The model under review builds one solid part; all positions refer to its coordinate system, in mm. Face numbers are marked on the shaded views. Coordinates: 2 decimals unless noted, no trailing zeros. Write each loop counter-clockwise with the first axis right and the second up, starting at its lowest first coordinate (ties: lowest second). Pieces come first, ordered by that corner, then holes. Notation, with made-up numbers: M 10.5,-24.5 L 23.5,-24.5 A28 ccw 23.5,6.5 Z; hole C 17,-18 d1. An arc over 180 degrees is marked long. Answer as a JSON object with one key per item and string values.
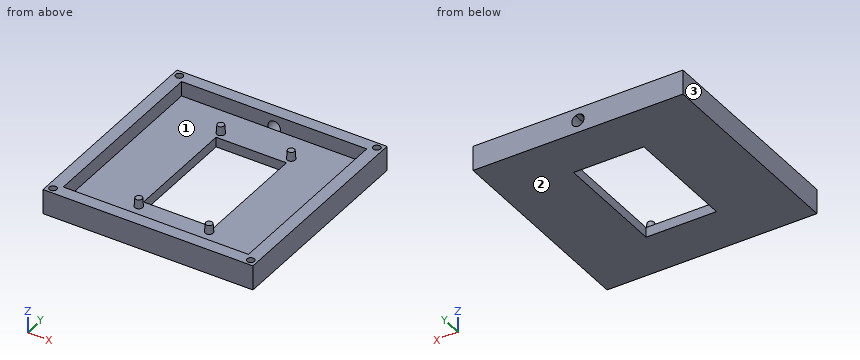
Autodesk Fusion 360 part; units mm, degrees
sketch "Sketch1" plane through (0, 0, 0) normal (0, 0, 1) x (1, 0, 0)
  line L0 (0, 0) -> (0, 75)
  line L1 (0, 75) -> (75, 75)
  line L2 (0, 0) -> (75, 0)
  line L3 (75, 0) -> (75, 75)
  line L4 (75, 75) -> (0, 75)
  line L5 (0, 75) -> (0, 0)
  line L6 (-5, -5) -> (80, -5)
  line L7 (80, -5) -> (80, 80)
  line L8 (80, 80) -> (-5, 80)
  line L9 (-5, 80) -> (-5, -5)
  line L10 (-5, -5) -> (80, -5)
  line L11 (80, -5) -> (80, 80)
  dimension "d1" = 75
  dimension "d2" = 75
  dimension "d3" = 85
extrude "Extrude1" add sketch "Sketch1" along normal blind 10
sketch "Sketch2" plane through (0, 0, 0) normal (0, 0, 1) x (1, 0, 0)
  line L0 (0, 0) -> (75, 0)
  line L1 (75, 0) -> (75, 75)
  line L2 (75, 75) -> (0, 75)
  line L3 (0, 75) -> (0, 0)
extrude "Extrude2" add sketch "Sketch2" along normal blind 4
sketch "Sketch3" plane through (0, 0, 4) normal (0, 0, 1) x (-1, 0, 0)
  line L0 (0, -75) -> (0, 0)
  line L1 (0, 0) -> (-75, 0)
  line L2 (-75, 0) -> (-75, -75)
  line L3 (-75, -75) -> (0, -75)
  line L4 (0, -75) -> (-75, 0)
  line L5 (0, 0) -> (-75, -75)
  line L6 (-37.5, -37.5) -> (-20.25, -37.5)
  line L7 (-37.5, -37.5) -> (-54.75, -37.5)
  line L8 (-20.25, -37.5) -> (-20.25, -66.5)
  line L9 (-54.75, -37.5) -> (-54.75, -8.5)
  line L10 (-20.25, -66.5) -> (-54.75, -66.5)
  line L11 (-54.75, -66.5) -> (-54.75, -8.5)
  line L12 (-54.75, -8.5) -> (-20.25, -8.5)
  line L13 (-20.25, -8.5) -> (-20.25, -66.5)
  line L14 (-37.5, -37.5) -> (-37.5, -60.5)
  line L15 (-37.5, -37.5) -> (-37.5, -14.5)
  line L16 (-37.5, -14.5) -> (-51.75, -14.5)
  line L17 (-37.5, -60.5) -> (-23.25, -60.5)
  line L18 (-23.25, -60.5) -> (-51.75, -60.5)
  line L19 (-51.75, -60.5) -> (-51.75, -14.5)
  line L20 (-51.75, -14.5) -> (-23.25, -14.5)
  line L21 (-23.25, -14.5) -> (-23.25, -60.5)
  dimension "d8" = 17.25
  dimension "d9" = 17.25
  dimension "d10" = 29
  dimension "d11" = 29
  dimension "d12" = 23
  dimension "d13" = 23
  dimension "d14" = 14.25
  dimension "d15" = 14.25
extrude "Extrude3" cut sketch "Sketch3" against normal blind 5 contours L4 L14 L17 L18 L21 | L4 L6 L21 | L5 L6 L21 | L5 L15 L20 L21 | L5 L7 L19 | L5 L14 L18 L19 | L4 L7 L19 | L4 L15 L16 L19 L20
sketch "Sketch4" plane through (0, 0, 4) normal (0, 0, 1) x (-1, 0, 0)
  line L0 (-51.75, -60.5) -> (-51.75, -14.5)
  line L1 (-51.75, -14.5) -> (-23.25, -14.5)
  line L2 (-23.25, -14.5) -> (-23.25, -60.5)
  line L3 (-23.25, -60.5) -> (-51.75, -60.5)
  line L4 (0, -75) -> (0, 0)
  line L5 (0, 0) -> (-75, 0)
  line L6 (-75, 0) -> (-75, -75)
  line L7 (-75, -75) -> (0, -75)
  line L8 (-75, 0) -> (0, -75)
  line L9 (-75, -75) -> (0, 0)
  line L10 (-37.5, -37.5) -> (-54.75, -37.5)
  line L11 (-54.75, -37.5) -> (-54.75, -8.5)
  line L12 (-54.75, -8.5) -> (-20.25, -8.5)
  line L13 (-20.25, -8.5) -> (-20.25, -66.5)
  line L14 (-20.25, -66.5) -> (-54.75, -66.5)
  line L15 (-54.75, -66.5) -> (-54.75, -8.5)
  line L16 (-54.75, -8.5) -> (-20.25, -8.5)
  line L17 (-20.25, -8.5) -> (-20.25, -66.5)
  line L18 (-20.25, -66.5) -> (-20.25, -63.5)
  line L19 (-20.25, -63.5) -> (-23.25, -63.5)
  circle A0 centre (-23.25, -63.5) radius 1.6
  line L20 (-54.75, -66.5) -> (-51.75, -66.5)
  line L21 (-51.75, -66.5) -> (-51.75, -63.5)
  circle A1 centre (-51.75, -63.5) radius 1.6
  line L22 (-20.25, -8.5) -> (-23.25, -8.5)
  line L23 (-23.25, -8.5) -> (-23.25, -11.5)
  circle A2 centre (-23.25, -11.5) radius 1.6
  line L24 (-54.75, -8.5) -> (-54.75, -11.5)
  line L25 (-54.75, -11.5) -> (-51.75, -11.5)
  circle A3 centre (-51.75, -11.5) radius 1.6
  dimension "d23" = 17.25
  dimension "d24" = 29
  dimension "d25" = 34.5
  dimension "d26" = 58
  dimension "d27" = 3
  dimension "d28" = 3
  dimension "d29" = 3.2
  dimension "d30" = 3
  dimension "d31" = 3
  dimension "d32" = 3.2
  dimension "d33" = 3
  dimension "d34" = 3
  dimension "d35" = 3.2
  dimension "d36" = 3
  dimension "d37" = 3
  dimension "d38" = 3.2
extrude "Extrude4" add sketch "Sketch4" along normal blind 3.5 draft -4 contours A1 | A0 | A2 | A3
sketch "Sketch5" plane through (0, 0, 10) normal (0, 0, 1) x (-1, 0, 0)
  line L0 (0, 0) -> (0, -75)
  line L1 (0, -75) -> (-75, -75)
  line L2 (-75, -75) -> (-75, 0)
  line L3 (-75, 0) -> (0, 0)
  line L4 (-80, 5) -> (-80, -80)
  line L5 (-80, -80) -> (5, -80)
  line L6 (5, -80) -> (5, 5)
  line L7 (5, 5) -> (-80, 5)
  line L8 (5, 5) -> (0, 0)
  line L9 (5, 0) -> (0, 5)
  circle A0 centre (2.5, 2.5) radius 1.5
  line L10 (-75, 0) -> (-80, 5)
  circle A1 centre (-77.5, 2.5) radius 1.5
  line L11 (-75, 5) -> (-80, 0)
  circle A2 centre (-77.5, -77.5) radius 1.5
  circle A3 centre (2.5, -77.5) radius 1.5
  dimension "d41" = 3
  dimension "d43" = 3
  dimension "d44" = 3
  dimension "d45" = 3
extrude "Extrude5" cut sketch "Sketch5" against normal blind 4 contours L8 L9 A0 | L8 L9 A0 | L10 A1 L11 | L10 A1 L11 | L8 L9 A0 | L8 L9 A0 | L10 A1 L11 | L10 A1 L11 | A2 | A3
sketch "Sketch6" plane through (0, 75, 0) normal (0, -1, 0) x (1, 0, 0)
  line L0 (0, 4) -> (75, 4)
  line L1 (75, 4) -> (75, 10)
  line L2 (75, 10) -> (0, 10)
  line L3 (0, 10) -> (0, 4)
  line L4 (75, 4) -> (0, 10)
  line L5 (0, 4) -> (75, 10)
  line L6 (38.5, 6.7) -> (36.5, 6.7)
  line L7 (36.5, 6.7) -> (36.5, 7.3)
  line L8 (36.5, 7.3) -> (38.5, 7.3)
  line L9 (38.5, 7.3) -> (38.5, 6.7)
  line L10 (38.5, 6.7) -> (36.5, 7.3) construction
  line L11 (36.5, 6.7) -> (38.5, 7.3) construction
  point P0 (37.5, 7)
extrude "Extrude6" cut sketch "Sketch6" against normal blind 5 contours L4 L5 L7 | L4 L5 L6 L7 L9 | L4 L5 L9 | L4 L5 L7 L8 L9
sketch "Sketch7" plane through (0, 80, 0) normal (0, 1, 0) x (-1, 0, 0)
  line L0 (-36.5, 7.3) -> (-36.5, 6.7)
  line L1 (-38.5, 6.7) -> (-38.5, 7.3)
  line L2 (-80, 0) -> (5, 0)
  line L3 (5, 0) -> (5, 10)
  line L4 (5, 10) -> (-80, 10)
  line L5 (-80, 10) -> (-80, 0)
  line L6 (5, 0) -> (-80, 10)
  line L7 (-80, 0) -> (5, 10)
  circle A0 centre (-37.5, 5) radius 2.5
  dimension "d50" = 5
extrude "Extrude7" cut sketch "Sketch7" against normal blind 5 contours L6 L7 A0 | L6 L7 A0 | L6 L7 A0 | L6 L7 A0
equation "d8 = ( 34.5 / 2 ) * 1 mm"
equation "d9 = ( 34.5 / 2 ) * 1 mm"
equation "d10 = ( 58 / 2 ) * 1 mm"
equation "d11 = ( 58 / 2 ) * 1 mm"
equation "d12 = ( 46 / 2 ) * 1 mm"
equation "d13 = ( 46 / 2 ) * 1 mm"
equation "d14 = ( 28.5 / 2 ) * 1 mm"
equation "d15 = ( 28.5 / 2 ) * 1 mm"
equation "d23 = ( 34.5 / 2 ) * 1 mm"
equation "d24 = ( 58 / 2 ) * 1 mm"
(1) For pin 1 Ø3 at (x, y) = (51, 64) entering from +Z; pin 2 Ø3.5 at (x, y) = (77.5, 77.5) entering from -Z; pin 3 Ø0.9 at (x, y) = (-2, 77) entering from +Z; pin 4 Ø22.5 at (x, y) = (40, 27) entering from +Z, all flat-tipped, find the tip position at first contact; note any pin that passes through.
Results list:
{"pin 1": "z = 7.5", "pin 2": "z = 0", "pin 3": "z = 6", "pin 4": "through"}
(2) Add section D-D on y = 67.5. Give the boundary of the cut face in (x, z).
Results list:
{"outline": "M -5,0 L 80,0 L 80,10 L 75,10 L 75,4 L 0,4 L 0,10 L -5,10 Z"}
(3) Wall thickness on line 1 along Y through (x, z) = (77.5, 6.85); line 2 along X through (y, z) = (27, 8.5): over which ranges is each line inside the solid? List them lowest first. Write a range as from..to.
Results list:
{"line 1": "-5..-4, -1..76, 79..80", "line 2": "-5..0, 75..80"}
(4) Add section C-C on x = 47. Give the boundary of the cut face in (y, z), and give its area (3 significant figures).
Results list:
{"outline": "M -5,0 L 14.5,0 L 14.5,4 L 0,4 L 0,10 L -5,10 Z; M 60.5,0 L 80,0 L 80,10 L 75,10 L 75,4 L 60.5,4 Z", "area": "216 mm²"}
(5) Draft analysis for pull direction X (two halves, no side actions). For the marked faces 1, 2 and 3, state which applies: released by +X, released by -X, zero draft, split by the parting line, or undercut.
Results list:
{"face 1": "undercut", "face 2": "zero draft", "face 3": "released by -X"}
(6) Add section A-A on x = 37.5. Give the boundary of the cut face in (y, z).
Results list:
{"outline": "M -5,0 L 14.5,0 L 14.5,4 L 0,4 L 0,10 L -5,10 Z; M 60.5,0 L 80,0 L 80,2.5 L 75,2.5 L 75,4 L 60.5,4 Z; M 75,7.5 L 80,7.5 L 80,10 L 75,10 Z"}
(7) Add section B-B on y = 30. Give the boundary of the cut face in (x, z).
Results list:
{"outline": "M -5,0 L 23.25,0 L 23.25,4 L 0,4 L 0,10 L -5,10 Z; M 51.75,0 L 80,0 L 80,10 L 75,10 L 75,4 L 51.75,4 Z"}
